The model under review builds one solid part; all positions refer to its coordinate system, in mm. A direction names the side the tool comes from. Coordinates: 2 decimals unless noted, no trailing zeros. Loops run counter-clockwise (first coordinate to the right, second up) from the corner with the lowest first, then second, coordinate; pieces in that order, holes last. Notation, with made-up numbers: M 70.5,11.5 L 102.5,11.5 A21 cw 102.5,48.5 Z; hole C -36.5,63.5 d1. An arc over 180 degrees is marked long. Return JSON: item names as keys, results as strings.
```python
from build123d import *

# Parameters (mm, degrees)
SKETCH1_R               = 10
BOSS_EXTRUDE1_DEPTH     = 12
SKETCH2_R               = 15
SKETCH2_R_2             = 10
BOSS_EXTRUDE2_DEPTH     = 6
CUT_EXTRUDE1_DEPTH      = 58.827329179
CIRPATTERN1_COUNT       = 4
SKETCH1_4_R             = 4.5
BOSS_EXTRUDE3_DEPTH     = 6
SKETCH1_5_R             = 4.5
SKETCH1_5_R_2           = 3.5
SKETCH1_5_R_3           = 2.5
BOSS_EXTRUDE4_DEPTH     = 2
CIRPATTERN2_COUNT       = 4
CHAMFER3_SIZE           = 3
SHELL1_T                = -1
CUT_EXTRUDE3_START      = -11
SKETCH9_R               = 11
CUT_EXTRUDE3_DEPTH      = 11
SKETCH10_R              = 11
CUT_EXTRUDE4_DEPTH      = 6
BOSS_EXTRUDE5_DEPTH     = 6
BOSS_EXTRUDE5_2_DEPTH   = 6
CUT_EXTRUDE7_DEPTH      = 60.363288319
CUT_EXTRUDE7_DEPTH_BACK = 60.363288319
SKETCH14_OUTSIDE_W      = 138.05
SKETCH14_OUTSIDE_H      = 42.912
CIRPATTERN5_COUNT       = 4
CUT_EXTRUDE8_DEPTH      = 59.787753827
CUT_EXTRUDE8_DEPTH_BACK = 59.787753827
SKETCH15_R              = 2.5


with BuildPart() as part:
    # Sketch1 → Boss-Extrude1 (new body)
    with BuildSketch(Plane(origin=(0, 0, 0), x_dir=(1, 0, 0), z_dir=(0, 1, 0))):
        with BuildLine():
            Line((24, 40), (-24, 40))
            Line((-24, 40), (-24, 32))
            ThreePointArc((-24, 32), (-26.343145751, 26.343145751), (-32, 24))
            Line((-32, 24), (-40, 24))
            Line((-40, 24), (-40, -24))
            Line((-40, -24), (-32, -24))
            ThreePointArc((-32, -24), (-26.343145751, -26.343145751), (-24, -32))
            Line((-24, -32), (-24, -40))
            Line((-24, -40), (24, -40))
            Line((24, -40), (24, -32))
            ThreePointArc((24, -32), (26.343145751, -26.343145751), (32, -24))
            Line((32, -24), (40, -24))
            Line((40, -24), (40, 24))
            Line((40, 24), (32, 24))
            ThreePointArc((32, 24), (26.343145751, 26.343145751), (24, 32))
            Line((24, 32), (24, 40))
        make_face()
        with Locations(Location((0, 0, 0), (0, 0, 270))):
            Circle(SKETCH1_R, mode=Mode.SUBTRACT)
    extrude(amount=BOSS_EXTRUDE1_DEPTH)

    # Sketch2 → Boss-Extrude2 (add)
    with BuildSketch(Plane(origin=(0, 12, 0), x_dir=(1, 0, 0), z_dir=(0, 1, 0))):
        with Locations(Location((0, 0, 0), (0, 0, 270))):
            Circle(SKETCH2_R)
        with Locations(Location((0, 0, 0), (0, 0, 270))):
            Circle(SKETCH2_R_2, mode=Mode.SUBTRACT)
    extrude(amount=BOSS_EXTRUDE2_DEPTH)

    # Sketch3 → Cut-Extrude1 (cut, through all)
    with BuildSketch(Plane(origin=(0, 12, 0), x_dir=(1, 0, 0), z_dir=(0, 1, 0))):
        with BuildLine():
            Line((21, -37), (-21, -37))
            Line((-21, -37), (-21, -32.313708499))
            Line((-21, -32.313708499), (-5.744900001, -17.0586085))
            ThreePointArc((-5.744900001, -17.0586085), (0, -18), (5.744900001, -17.0586085))
            Line((5.744900001, -17.0586085), (21, -32.313708499))
            Line((21, -32.313708499), (21, -37))
        make_face()
    cut_extrude1 = extrude(amount=-CUT_EXTRUDE1_DEPTH, mode=Mode.SUBTRACT)

    # CirPattern1: Cut-Extrude1 ×4 about axis
    cirpattern1_axis = Axis((0, 0, 0), (0, 1, 0))
    for i in range(1, CIRPATTERN1_COUNT):
        add(cut_extrude1.rotate(cirpattern1_axis, i * 360 / CIRPATTERN1_COUNT), mode=Mode.SUBTRACT)

    # Sketch1<4> → Boss-Extrude3 (add)
    with BuildSketch(Plane(origin=(0, 0, 0), x_dir=(1, 0, 0), z_dir=(0, 1, 0))):
        with BuildLine():
            Line((-24, 32), (-24, 40))
            Line((-24, 40), (-40, 40))
            Line((-40, 40), (-40, 24))
            Line((-40, 24), (-32, 24))
            ThreePointArc((-32, 24), (-26.343145751, 26.343145751), (-24, 32))
        make_face()
        with Locations(Location((-32, 32, 0), (0, 0, 270))):
            Circle(SKETCH1_4_R, mode=Mode.SUBTRACT)
    boss_extrude3 = extrude(amount=BOSS_EXTRUDE3_DEPTH)

    # Sketch1<5> → Boss-Extrude4 (add)
    # profile 1 of 3: a face of its own
    with BuildSketch(Plane(origin=(0, 0, 0), x_dir=(1, 0, 0), z_dir=(0, 1, 0))):
        with Locations(Location((-32, 32, 0), (0, 0, 270))):
            Circle(SKETCH1_5_R)
        with Locations((-32, 32)):
            Circle(SKETCH1_5_R_2, mode=Mode.SUBTRACT)
    # profile 2 of 3: a face of its own
    with BuildSketch(Plane(origin=(0, 0, 0), x_dir=(1, 0, 0), z_dir=(0, 1, 0))):
        with Locations((-32, 32)):
            Circle(SKETCH1_5_R_2)
        with Locations((-32, 32)):
            Circle(SKETCH1_5_R_3, mode=Mode.SUBTRACT)
    # profile 3 of 3: a face of its own
    with BuildSketch(Plane(origin=(0, 0, 0), x_dir=(1, 0, 0), z_dir=(0, 1, 0))):
        with Locations((-32, 32)):
            Circle(SKETCH1_5_R_3)
    boss_extrude4 = extrude(amount=BOSS_EXTRUDE4_DEPTH)

    # CirPattern2: Boss-Extrude3, Boss-Extrude4 ×4 about axis
    cirpattern2_axis = Axis((0, 0, 0), (0, 1, 0))
    add([boss_extrude3.rotate(cirpattern2_axis, i * 360 / CIRPATTERN2_COUNT) for i in range(1, CIRPATTERN2_COUNT)])
    add([boss_extrude4.rotate(cirpattern2_axis, i * 360 / CIRPATTERN2_COUNT) for i in range(1, CIRPATTERN2_COUNT)])

    # Chamfer3
    chamfer3_edges = [part.edges().sort_by_distance(p)[0] for p in [
        (-40, 3, -40),
        (40, 3, -40),
        (40, 3, 40),
        (-40, 3, 40),
    ]]
    chamfer(chamfer3_edges, length=CHAMFER3_SIZE)

    # Shell1
    shell1_openings = [part.faces().sort_by_distance(p)[0] for p in [
        (0, 0, -28.947670916),
    ]]
    offset(amount=SHELL1_T, openings=shell1_openings, kind=Kind.INTERSECTION)

    # Sketch9 → Cut-Extrude3 (cut)
    with BuildSketch(Plane.XZ.offset(CUT_EXTRUDE3_START)):
        with Locations(Location((0, 0, 0), (0, 0, 90))):
            Circle(SKETCH9_R)
        with BuildLine():
            Line((22, 38), (-22, 38))
            Line((-22, 38), (-22, 31.899494937))
            Line((-22, 31.899494937), (-6.004703682, 15.904198618))
            ThreePointArc((-6.004703682, 15.904198618), (0, 17), (6.004703682, 15.904198618))
            Line((6.004703682, 15.904198618), (22, 31.899494937))
            Line((22, 31.899494937), (22, 38))
        make_face()
        with BuildLine():
            Line((-38, 22), (-38, -22))
            Line((-38, -22), (-31.899494937, -22))
            Line((-31.899494937, -22), (-15.904198618, -6.004703682))
            ThreePointArc((-15.904198618, -6.004703682), (-17, 0), (-15.904198618, 6.004703682))
            Line((-15.904198618, 6.004703682), (-31.899494937, 22))
            Line((-31.899494937, 22), (-38, 22))
        make_face()
        with BuildLine():
            Line((-22, -38), (22, -38))
            Line((22, -38), (22, -31.899494937))
            Line((22, -31.899494937), (6.004703682, -15.904198618))
            ThreePointArc((6.004703682, -15.904198618), (0, -17), (-6.004703682, -15.904198618))
            Line((-6.004703682, -15.904198618), (-22, -31.899494937))
            Line((-22, -31.899494937), (-22, -38))
        make_face()
        with BuildLine():
            Line((38, -22), (38, 22))
            Line((38, 22), (31.899494937, 22))
            Line((31.899494937, 22), (15.904198618, 6.004703682))
            ThreePointArc((15.904198618, 6.004703682), (17, 0), (15.904198618, -6.004703682))
            Line((15.904198618, -6.004703682), (31.899494937, -22))
            Line((31.899494937, -22), (38, -22))
        make_face()
    extrude(amount=CUT_EXTRUDE3_DEPTH, mode=Mode.SUBTRACT)

    # Sketch10 → Cut-Extrude4 (cut)
    with BuildSketch(Plane.XZ.offset(-11)):
        Circle(SKETCH10_R)
    extrude(amount=-CUT_EXTRUDE4_DEPTH, mode=Mode.SUBTRACT)

    # Sketch15 → Cut-Extrude8 (cut, two sides: drawn at the far end of the back side and taken through both)
    with BuildSketch(Plane(origin=(0, 2, 0), x_dir=(1, 0, 0), z_dir=(0, 1, 0)).offset(-CUT_EXTRUDE8_DEPTH_BACK)):
        with Locations(Location((-32, -32, 0), (0, 0, 270))):
            Circle(SKETCH15_R)
        with Locations(Location((-32, 32, 0), (0, 0, 270))):
            Circle(SKETCH15_R)
        with Locations(Location((32, 32, 0), (0, 0, 270))):
            Circle(SKETCH15_R)
        with Locations(Location((32, -32, 0), (0, 0, 270))):
            Circle(SKETCH15_R)
    extrude(amount=CUT_EXTRUDE8_DEPTH + CUT_EXTRUDE8_DEPTH_BACK, mode=Mode.SUBTRACT)


with BuildPart() as body_2:
    # Sketch12 → Boss-Extrude5 (new body)
    with BuildSketch(Plane(origin=(0, 12, 0), x_dir=(1, 0, 0), z_dir=(0, 1, 0))):
        with BuildLine():
            Line((-6.464466094, -13.535533906), (-20.606601718, -27.67766953))
            Line((-20.606601718, -27.67766953), (-21.66726189, -26.617009358))
            Line((-21.66726189, -26.617009358), (-7.838951938, -12.788699407))
            ThreePointArc((-7.838951938, -12.788699407), (-7.16145113, -13.180046195), (-6.464466094, -13.535533906))
        make_face()
    extrude(amount=BOSS_EXTRUDE5_DEPTH)


with BuildPart() as body_3:
    # Sketch12 → Boss-Extrude5 2 (new body)
    with BuildSketch(Plane(origin=(0, 12, 0), x_dir=(1, 0, 0), z_dir=(0, 1, 0))):
        with BuildLine():
            Line((-13.535533906, -6.464466094), (-27.67766953, -20.606601718))
            Line((-27.67766953, -20.606601718), (-26.617009358, -21.66726189))
            Line((-26.617009358, -21.66726189), (-12.788699407, -7.838951938))
            ThreePointArc((-12.788699407, -7.838951938), (-13.180046195, -7.16145113), (-13.535533906, -6.464466094))
        make_face()
    extrude(amount=BOSS_EXTRUDE5_2_DEPTH)


with BuildPart() as cut_extrude7_tool:
    # Sketch14 outside → Cut-Extrude7 (new, two sides: drawn at the far end of the back side and taken through both)
    with BuildSketch(Plane(origin=(0, 0, 0), x_dir=(0.7071067811865476, 0, -0.7071067811865476), z_dir=(0.7071067811865476, 0, 0.7071067811865476)).offset(-CUT_EXTRUDE7_DEPTH_BACK)):
        with Locations((0, 9)):
            Rectangle(SKETCH14_OUTSIDE_W, SKETCH14_OUTSIDE_H)
        Polygon((-14.142135624, 16), (-34.142135624, 12), (-14.142135624, 12), align=None, mode=Mode.SUBTRACT)
    extrude(amount=CUT_EXTRUDE7_DEPTH + CUT_EXTRUDE7_DEPTH_BACK)


with BuildPart() as body_3_1:
    add(body_3.part)

    # Cut-Extrude7: cut by cut_extrude7_tool
    add(cut_extrude7_tool.part, mode=Mode.SUBTRACT)


with BuildPart() as body_2_1:
    add(body_2.part)

    # Cut-Extrude7: cut by cut_extrude7_tool
    add(cut_extrude7_tool.part, mode=Mode.SUBTRACT)


with BuildPart() as cirpattern5_1:
    # CirPattern5: pattern copy
    add(body_2_1.part.rotate(Axis((0, 0, 0), (0, 1, 0)), 1 * 360 / CIRPATTERN5_COUNT))


with BuildPart() as cirpattern5_2:
    # CirPattern5: pattern copy
    add(body_2_1.part.rotate(Axis((0, 0, 0), (0, 1, 0)), 2 * 360 / CIRPATTERN5_COUNT))


with BuildPart() as cirpattern5_3:
    # CirPattern5: pattern copy
    add(body_2_1.part.rotate(Axis((0, 0, 0), (0, 1, 0)), 3 * 360 / CIRPATTERN5_COUNT))


with BuildPart() as cirpattern5_4:
    # CirPattern5: pattern copy
    add(body_3_1.part.rotate(Axis((0, 0, 0), (0, 1, 0)), 1 * 360 / CIRPATTERN5_COUNT))


with BuildPart() as cirpattern5_5:
    # CirPattern5: pattern copy
    add(body_3_1.part.rotate(Axis((0, 0, 0), (0, 1, 0)), 2 * 360 / CIRPATTERN5_COUNT))


with BuildPart() as cirpattern5_6:
    # CirPattern5: pattern copy
    add(body_3_1.part.rotate(Axis((0, 0, 0), (0, 1, 0)), 3 * 360 / CIRPATTERN5_COUNT))


with BuildPart() as cirpattern5_5_1:
    add(cirpattern5_5.part)

    # Combine1: union CirPattern5_3, body 2, CirPattern5_1, CirPattern5_6, body 3, CirPattern5_4, part, CirPattern5_2
    add(cirpattern5_3.part)
    add(body_2_1.part)
    add(cirpattern5_1.part)
    add(cirpattern5_6.part)
    add(body_3_1.part)
    add(cirpattern5_4.part)
    add(part.part)
    add(cirpattern5_2.part)


solid = cirpattern5_5_1.part
```
1. Machinability: for faces 4 (the face through (11.87, 13.53, -18.94)), 5 (the face through (26.406, 8.958, -26.281)), 6 (the face through (-18.94, 13.53, 11.87)), 7 (the face through (-34, 2, -30)), 8 (the face through (-26.281, 8.958, -26.406)), which of the approach directions +Z, -Z, +X, -X, +Y, -Y give a long, thin tool a straight path to every point of the face, cutting with its end or side? Answer none if there is none.
Check values:
{"face 4": "-Z, +Y", "face 5": "-Z, +X, +Y", "face 6": "-X, +Y", "face 7": "+Y", "face 8": "-Z, -X, +Y"}
2. Add section B-B on x = 0. Give the boundary of the cut face in (y, z), plus the area to 3 significant figures.
Check values:
{"outline": "M 0,-40 L 12,-40 L 12,-37 L 11,-37 L 11,-39 L 0,-39 Z; M 0,39 L 11,39 L 11,37 L 12,37 L 12,40 L 0,40 Z; M 11,-18 L 12,-18 L 12,-15 L 18,-15 L 18,-10 L 17,-10 L 17,-14 L 11,-14 Z; M 11,14 L 17,14 L 17,10 L 18,10 L 18,15 L 12,15 L 12,18 L 11,18 Z", "area": "56.0 mm²"}
3. Insertion check: pin 1 Ø10 at (x, z) = (2.5, -17) entering from -Y; pin 2 Ø9 at (x, z) = (34, 33.5) entering from -Y; pin 3 Ø1.5 at (x, y) = (-9.5, 14) entering from +Z. Each pin has a flat end and moves straight along its axis. Give the tip position at first contact, or say it passes through.
Check values:
{"pin 1": "y = 11", "pin 2": "y = 1", "pin 3": "z = 17.32"}
4. Add section A-A on z = 0. Give the boundary of the cut face in (x, y).
Check values:
{"outline": "M -40,0 L -39,0 L -39,11 L -37,11 L -37,12 L -40,12 Z; M -18,11 L -14,11 L -14,17 L -10,17 L -10,18 L -15,18 L -15,12 L -18,12 Z; M 10,17 L 14,17 L 14,11 L 18,11 L 18,12 L 15,12 L 15,18 L 10,18 Z; M 37,11 L 39,11 L 39,0 L 40,0 L 40,12 L 37,12 Z"}
5. The part is to be moulded in two halves that separate along Z. For faces 1 (the face through (-11.87, 13.53, -18.94)), 2 (the face through (13.479, 11.507, -24.793)), 3 (the face through (-40, 5, -1)), say which applies: released by +Z, released by -Z, zero draft, split by the parting line, or undercut.
Check values:
{"face 1": "released by -Z", "face 2": "undercut", "face 3": "zero draft"}
6. To check wall thickness, follow line 1 (X direction, y = 10.5, z = -35.5); line 2 (Z direction, x = 4.5, y = 4.5); line 3 (Z direction, x = 0, y = 12.95). State the ranges of each line that lie inside material, in increasing order.
Check values:
{"line 1": "-24 to -23, 23 to 24", "line 2": "-40 to -39, 39 to 40", "line 3": "-15 to -14, 14 to 15"}
